The model under review builds one solid part; all positions refer to its coordinate system, in mm. Face numbers are marked on the shaded views. Round coordinates to 2 decimals unless told otherwise and drop trailing zeros. Order: outer loops, then holes, each group sorted by start corner. A loop starts at its lowest first (then second) coordinate and runs counter-clockwise, first axis right, second up. Notation, with made-up numbers: (72.5, 9.5) -> (115.5, 9.5) arc R31 ccw to (115.5, 47.5) -> close; hole circle Ø2 at (-38, 64.5). An arc over 180 degrees is marked (long way). Use a Markdown table: item, result. Add a question column.
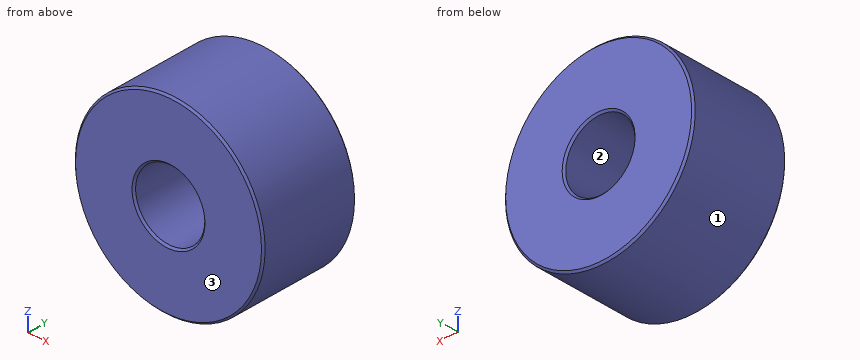
```python
from build123d import *

# Parameters (mm, degrees)
F0_R     = 63.833527
F0_R_2   = 23.253749
F1_DEPTH = 68.326
F2_SIZE  = 1.27


with BuildPart() as f1:
    # F0 (on Front) → F1 (new body)
    with BuildSketch(Plane.XZ):
        Circle(F0_R)
        Circle(F0_R_2, mode=Mode.SUBTRACT)
    extrude(amount=F1_DEPTH)

    # F2
    f2_edges = [f1.edges().sort_by_distance(p)[0] for p in [
        (23.253749, -34.163, 0),
        (-23.253749, 0, 0),
        (-23.253749, -68.326, 0),
        (-63.833527, -68.326, 0),
        (-63.833527, 0, 0),
    ]]
    chamfer(f2_edges, length=F2_SIZE)


solid = f1.part
```
Q1. For pin 1 (1.5 mm diameter, centred on x = 12, z = -50.5, fed in from +Y); pin 2 (12 mm diameter, centred on y = -41.5, z = 35, fed in from -X); pin 3 (10 mm diameter, centred on y = -56.5, z = 49, fed in from -X); pin 4 (2 mm diameter, centred on y = -8.5, z = 38, fed in from -X), all flat-tipped, find the tip position at first contact; note any pin that passes through.
Q2. Add section C-C, the plane y = -24. Give the boundary of the cut face in (x, z).
Q3. Add section B-B, the plane x = 0. Give the boundary of the cut face in (y, z), then the cut area to 3 significant figures.
Q4. To check wall thickness, follow line 1 along Z through (x, y) = (0, -51); line 2 along X through (y, z) = (-43, -4.5); line 3 along Z through (x, y) = (-7.5, -16). State the ranges of each line that lie inside material, in increasing order.
Q5. Add section A-A, the plane z = 0. Give the boundary of the cut face in (x, y).
Q6. Draft analysis for pull direction Z (two halves, no side actions). For the marked faces 1, 2 and 3, state which applies: released by +Z, released by -Z, zero draft, split by the parting line, or undercut.
Return value:
| question | item | result |
|---|---|---|
| 1 | pin 1 | y = 0 |
| 1 | pin 2 | x = -56.87 |
| 1 | pin 3 | x = -46.25 |
| 1 | pin 4 | x = -52.02 |
| 2 | outline | circle Ø127.67 at (0, 0); hole circle Ø46.51 at (0, 0) |
| 3 | outline | (-68.33, -62.56) -> (-67.06, -63.83) -> (-1.27, -63.83) -> (0, -62.56) -> (0, -24.52) -> (-1.27, -23.25) -> (-67.06, -23.25) -> (-68.33, -24.52) -> close; (-68.33, 24.52) -> (-67.06, 23.25) -> (-1.27, 23.25) -> (0, 24.52) -> (0, 62.56) -> (-1.27, 63.83) -> (-67.06, 63.83) -> (-68.33, 62.56) -> close |
| 3 | area | 5,540 mm² |
| 4 | line 1 | -63.83 to -23.25, 23.25 to 63.83 |
| 4 | line 2 | -63.67 to -22.81, 22.81 to 63.67 |
| 4 | line 3 | -63.39 to -22.01, 22.01 to 63.39 |
| 5 | outline | (-63.83, -67.06) -> (-62.56, -68.33) -> (-24.52, -68.33) -> (-23.25, -67.06) -> (-23.25, -1.27) -> (-24.52, 0) -> (-62.56, 0) -> (-63.83, -1.27) -> close; (23.25, -67.06) -> (24.52, -68.33) -> (62.56, -68.33) -> (63.83, -67.06) -> (63.83, -1.27) -> (62.56, 0) -> (24.52, 0) -> (23.25, -1.27) -> close |
| 6 | face 1 | split by the parting line |
| 6 | face 2 | undercut |
| 6 | face 3 | zero draft |
